Input: part model. Units: mm. Frame: model coordinates. A direction names the side the tool comes from. Coordinates: 2 decimals unless noted, no trailing zeros. Loops run counter-clockwise (first coordinate to the right, second up) from the corner with the lowest first, then second, coordinate; pieces in that order, holes last.
Item 1: Reachability of faces 4 (the cylindrical face through (-13.887, -10.648, 8.58)), 5 (the cylindrical face through (-19.583, -8.12, 3.55)) from +Z, -Z, +X, -X, +Y, -Y: full face, straight path, thin tool, end or side. Return the list, or none.
Item 2: Section C-C on z = 6. Return loops of the section in (x, y), and give its area (3 significant figures).
Item 3: Section A-A on x = 0. Return loops of the section in (y, z), and give its area (3 significant figures).
Item 4: Contact query for flat-ended pins moving along their axis: P1, Ø2, axis at x = 15.5, z = 3.5, coming from the -Y side; P2, Ø4, axis at y = 13, z = 3.5, coming from the -X side; P3, Ø4, axis at y = -7.5, z = 6.5, coming from the +X side. Output: stop coordinate, or through.
Item 5: Pull-direction query (X, two-part tool) for faces 1 (the flat face through (-3, 17.4, 7.2)), 2 (the cylindrical face through (-3.411, 25.977, 4.93)), 3 (the flat face through (-0.1, 21.5, 0)); classes: released by +X, released by -X, zero draft, split by the parting line, or undercut.
Item 6: Ray query, line 1 along X through (y, z) = (0.5, 4.75); line 2 along Y through (x, z) = (16, 6); line 3 along X through (y, z) = (18, 3.5). Return the intervals inside material, ascending.
```python
from build123d import *

# Parameters (mm, degrees)
SKETCH1_R           = 26.2
SKETCH1_R_2         = 1.6
SKETCH1_R_3         = 17.5
BOSS_EXTRUDE1_DEPTH = 10
SKETCH2_R           = 21.2
CUT_EXTRUDE1_DEPTH  = 7.2


with BuildPart() as part:
    # Sketch1 → Boss-Extrude1 (new body)
    with BuildSketch(Plane.XY):
        Circle(SKETCH1_R)
        with Locations((17.349171734, 16.10572211)):
            Circle(SKETCH1_R_2, mode=Mode.SUBTRACT)
        with Locations((16.10572211, -17.349171734)):
            Circle(SKETCH1_R_2, mode=Mode.SUBTRACT)
        with Locations((-16.10572211, 17.349171734)):
            Circle(SKETCH1_R_2, mode=Mode.SUBTRACT)
        with Locations((-17.349171734, -16.10572211)):
            Circle(SKETCH1_R_2, mode=Mode.SUBTRACT)
        Circle(SKETCH1_R_3, mode=Mode.SUBTRACT)
    extrude(amount=BOSS_EXTRUDE1_DEPTH)

    # Sketch2 → Cut-Extrude1 (cut)
    with BuildSketch(Plane(origin=(0, 0, 0), x_dir=(-1, 0, 0), z_dir=(0, 0, -1))):
        Circle(SKETCH2_R)
    extrude(amount=-CUT_EXTRUDE1_DEPTH, mode=Mode.SUBTRACT)


solid = part.part
```
Results found:
1. face 4: +Z, -Z
1. face 5: -Z
2. outline: circle Ø52.4 at (0, 0); hole circle Ø42.4 at (0, 0); hole circle Ø3.2 at (-17.35, -16.11); hole circle Ø3.2 at (-16.11, 17.35); hole circle Ø3.2 at (16.11, -17.35); hole circle Ø3.2 at (17.35, 16.11)
2. area: 712 mm2
3. outline: (-26.2, 0) - (-21.2, 0) - (-21.2, 7.2) - (-17.5, 7.2) - (-17.5, 10) - (-26.2, 10) - close; (17.5, 7.2) - (21.2, 7.2) - (21.2, 0) - (26.2, 0) - (26.2, 10) - (17.5, 10) - close
3. area: 121 mm2
4. P1: stops at y = -21.82
4. P2: stops at x = -23.78
4. P3: stops at x = 25.62
5. face 1: undercut
5. face 2: split by the parting line
5. face 3: zero draft
6. line 1: x = -26.2 to -21.19, 21.19 to 26.2
6. line 2: y = -20.75 to -18.95, -15.75 to -13.91, 13.91 to 15.25, 16.97 to 20.75
6. line 3: x = -19.04 to -17.57, -14.64 to -11.2, 11.2 to 19.04
